Autodesk Fusion 360 part; units mm, degrees
sketch "Sketch1" plane through (0, 0, 0) normal (0, 0, 1) x (1, 0, 0) in component "ADAPTERI2"
  circle A0 centre (0, 0) radius 15
  dimension "d3" = 30
extrude "Extrude1" add sketch "Sketch1" along normal blind 50 in component "ADAPTERI2"
sketch "Sketch2" plane through (-0.004, -0.0691, 50) normal (0, 0, 1) x (-1, 0, 0) in component "ADAPTERI2"
  circle A0 centre (-0.004, -0.0691) radius 15
  line L0 (-4.5, 2.5) -> (4.5, 2.5)
  line L1 (4.5, 2.5) -> (4.5, -2.5)
  line L2 (4.5, -2.5) -> (-4.5, -2.5)
  line L3 (-4.5, -2.5) -> (-4.5, 2.5)
  line L4 (-4.5, 2.5) -> (4.5, -2.5) construction
  line L5 (4.5, 2.5) -> (-4.5, -2.5) construction
  dimension "d6" = 9
  dimension "d7" = 5
extrude "Extrude2" cut sketch "Sketch2" against normal blind 10 contours L0 L1 L2 L3 in component "ADAPTERI2"
sketch "Sketch3" plane through (-0.2192, -4.1274, 0) normal (0, 0, -1) x (1, 0, 0) in component "ADAPTERI2"
  circle A0 centre (0.2192, -4.1274) radius 15
  line L0 (0.3727, -11.0539) -> (6.2945, -7.4577)
  line L1 (6.2945, -7.4577) -> (6.1409, -0.5312)
  line L2 (6.1409, -0.5312) -> (0.0656, 2.7991)
  line L3 (0.0656, 2.7991) -> (-5.8561, -0.7971)
  line L4 (-5.8561, -0.7971) -> (-5.7026, -7.7236)
  line L5 (-5.7026, -7.7236) -> (0.3727, -11.0539)
  point P0 (0.2192, -4.1274)
  dimension "d10" = 6
extrude "Extrude3" cut sketch "Sketch3" against normal blind 20 contours L0 L1 L2 L3 L4 L5 in component "ADAPTERI2"
move_face "OffsetFaces1" offset -5 1 faces at (14.9255, -1.4935, 16.6667) in component "ADAPTERI2"
component "ADAPTERI2" placed x (1, 0, 0) y (0, 1, 0) z (0, 0, 1) at (0, 0, 0)
Read the model definition and answer for the solid it produces. Units are mm, in the model's axes. A direction names the side the tool comes from. Give positions to 0.01 mm unless a question says otherwise; leave off trailing zeros. Order: outer loops, then holes, each group sorted by start corner. A loop starts at its lowest first (then second) coordinate and runs counter-clockwise, first axis right, second up. Notation, with made-up numbers: (67, 34.5) -> (79, 34.5) arc R24 cw to (79, 64.5) -> close; hole circle Ø8 at (75, 83). An arc over 180 degrees is marked (long way). One line per item, written item: value. Start each with the question number.
(1) A tool of negligible diameter and unlimited length cuts with its end or side. For faces 4 (the flat face through (-2.927, 5.238, 9.86)), 5 (the flat face through (-4.504, 0, 45)), 6 (the flat face through (0, -4, 50)), from which of +Z, -Z, +X, -X, +Y, -Y can it reach the whole face along a straight path? Write none if from no direction.
(2) The part is cut by section B-B (x = -3.25). Determine the outline of the cut face in (y, z).
(3) Straight lines are drawn through the part: L1, parallel to X at y = -6.5, z = 19.5; L2, parallel to Y at x = -3, z = 6; L3, parallel to Z at x = 1, y = -3.25. For each, find the intervals that lie inside material, in ascending order.
(4) The part is cut by section C-C (y = 0). Determine the outline of the cut face in (x, z).
(5) Flat-ended cylindrical pins translate along their axes: P1, Ø2.5, axis at x = -1.5, z = 44.5, coming from the -Y side; P2, Ø2, axis at x = -4, y = 0, coming from the -Z side; P3, Ø4, axis at x = -5.5, z = 25.5, coming from the -Y side. Find the tip coordinate at first contact, or state that the pin passes through.
(6) The part is cut by section A-A (z = 42). Determine the outline of the cut face in (x, y), and give its area (3 significant figures).
(7) The part is cut by section D-D (z = 26.5). Determine the outline of the cut face in (x, y), and give its area (3 significant figures).
(8) For a pull along Y with two mould halves and no side action, classify faces 1 (the flat face through (0, -2.569, 45)), 2 (the cylindrical face through (-2.17, 9.76, 24.65)), 3 (the flat face through (4, 5, 0)) as released by +Y, released by -Y, zero draft, split by the parting line, or undercut.
Taken from the geometry:
1. face 4: -Z
1. face 5: +Z
1. face 6: +Z, +X, -X, +Y, -Y
2. outline: (-9.46, 0) -> (-5.05, 0) -> (-5.05, 20) -> (5.06, 20) -> (5.06, 0) -> (9.46, 0) -> (9.46, 50) -> (2.43, 50) -> (2.43, 40) -> (-2.57, 40) -> (-2.57, 50) -> (-9.46, 50) -> close
3. L1: -7.6 to -0.86, 0.62 to 7.6
3. L2: -9.54 to -5.2, 5.2 to 9.54
3. L3: 20 to 50
4. outline: (-10, 0) -> (-6, 0) -> (-6, 20) -> (6, 20) -> (6, 0) -> (10, 0) -> (10, 50) -> (4.5, 50) -> (4.5, 40) -> (-4.5, 40) -> (-4.5, 50) -> (-10, 50) -> close
5. P1: y = -10
5. P2: z = 20
5. P3: y = -9.37
6. outline: circle Ø20 at (0, 0); hole (-4.5, -2.57) -> (4.5, -2.57) -> (4.5, 2.43) -> (-4.5, 2.43) -> close
6. area: 269 mm^2
7. outline: circle Ø20 at (0, 0)
7. area: 314 mm^2
8. face 1: undercut
8. face 2: split by the parting line
8. face 3: zero draft
